```python
from build123d import *

# Parameters (mm, degrees)
F1_DEPTH = 12.7


with BuildPart() as f1:
    # F0 (on Front) → F1 (new body)
    with BuildSketch(Plane.XZ):
        with BuildLine():
            Line((5.500342, -28.573128), (16.227658, -9.978257))
            Line((16.227658, -9.978257), (16.76142, -9.053028))
            ThreePointArc((16.76142, -9.053028), (0.502926, 19.04336), (-17.215894, -8.155703))
            Line((-17.215894, -8.155703), (-15.728529, -10.74783))
            Line((-15.728529, -10.74783), (-5.507707, -28.560326))
            ThreePointArc((-5.507707, -28.560326), (-0.007385, -31.749996), (5.500342, -28.573128))
        make_face()
        with BuildLine():
            ThreePointArc((0, -12.7), (-8.980256, 8.980256), (12.7, 0))
            ThreePointArc((12.7, 0), (8.980256, -8.980256), (0, -12.7))
        make_face(mode=Mode.SUBTRACT)
    extrude(amount=-F1_DEPTH)


solid = f1.part
```
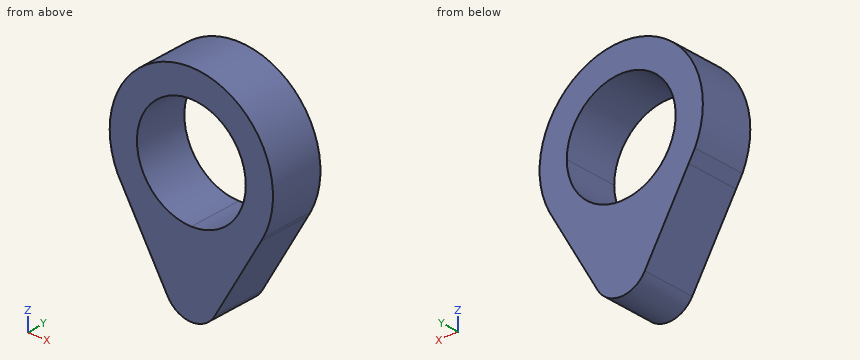
Geometry: final body of the model. Coordinates: model frame, mm. Coordinates: 2 decimals unless noted, no trailing zeros. Order: outer loops, then holes, each group sorted by start corner. A loop starts at its lowest first (then second) coordinate and runs counter-clockwise, first axis right, second up. Notation, with made-up numbers: M 12.25,-25 L 61.25,-25 A17 cw 61.25,-4 Z; hole C 68,40 d2. An arc over 180 degrees is marked long. Answer as CSV lines item,"result".
Q1. Section C-C on z = 2.5. Return the cut outline in (x, y).
Answers:
outline,"M -18.89,0 L -12.45,0 L -12.45,12.7 L -18.89,12.7 Z; M 12.45,0 L 18.89,0 L 18.89,12.7 L 12.45,12.7 Z"
Q2. Line query: probe 1 along Z at (x, y) = (-10, 0.75); probe 2 along Z at (x, y) = (7, 11); probe 3 along X at (y, z) = (7, -1). Output: solid intervals per line, ascending. Write a range as [from, to].
Answers:
probe 1,"z = [-20.73, -7.83], [7.83, 16.21]"
probe 2,"z = [-25.97, -10.6], [10.6, 17.72]"
probe 3,"x = [-19.02, -12.66], [12.66, 19.02]"
Q3. Section A-A on y = 3.25. Return the cut outline in (x, z).
Answers:
outline,"M -17.22,-8.16 L -15.73,-10.75 L -5.51,-28.56 A6.35 ccw 5.5,-28.57 L 16.23,-9.98 L 16.76,-9.05 A19.05 ccw long Z; hole C 0,0 d25.4"
Q4. Section B-B on x = 3. Return the cut outline in (y, z).
Answers:
outline,"M 0,-31 L 12.7,-31 L 12.7,-12.34 L 0,-12.34 Z; M 0,12.34 L 12.7,12.34 L 12.7,18.81 L 0,18.81 Z"
Q5. Section D-D on x = -14. Return the cut outline in (y, z).
Answers:
outline,"M 0,-13.76 L 12.7,-13.76 L 12.7,12.92 L 0,12.92 Z"
Q6. First-contact query: P1, Ø2, axis at x = -8.5, y = 9.5, coming from the +Z side; P2, Ø6, axis at x = -10, y = 6.5, coming from the +Z side; P3, Ø2, axis at x = 7, y = 6.5, coming from the +Z side. Flat tips, straight axial feed; report the tip coordinate or a pass-through.
Answers:
P1,"stops at z = 17.51"
P2,"stops at z = 17.72"
P3,"stops at z = 18.08"
